```python
from build123d import *

# Parameters (mm, degrees)
SKETCH1_R           = 4.5
BOSS_EXTRUDE1_DEPTH = 2.4
SKETCH2_R           = 0.5
CUT_EXTRUDE1_DEPTH  = 0.5


with BuildPart() as part:
    # Sketch1 → Boss-Extrude1 (new body)
    with BuildSketch(Plane.XY):
        Circle(SKETCH1_R)
    extrude(amount=BOSS_EXTRUDE1_DEPTH)

    # Sketch2 → Cut-Extrude1 (cut)
    with BuildSketch(Plane(origin=(0, 0, 0), x_dir=(-1, 0, 0), z_dir=(0, 0, -1))):
        with Locations((2, 0.068183801)):
            Circle(SKETCH2_R)
        with Locations((-2, -0.055218249)):
            Circle(SKETCH2_R)
    extrude(amount=-CUT_EXTRUDE1_DEPTH, mode=Mode.SUBTRACT)


solid = part.part
```
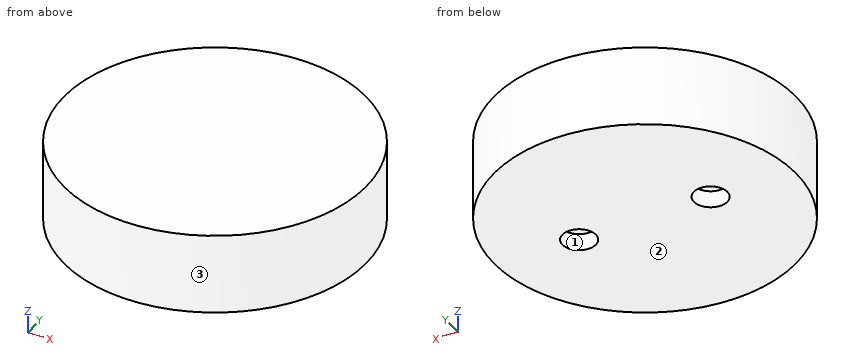
Read the model definition and answer for the solid it produces. Units are mm, in the model's axes. Face numbers are marked on the shaded views. Give positions to 0.01 mm unless a question says otherwise; leave off trailing zeros. Write each loop counter-clockwise with the first axis right and the second up, starting at its lowest first coordinate (ties: lowest second). Pieces come first, ordered by that corner, then holes. Notation, with made-up numbers: (74, -20) - (102, -20) arc R28 ccw to (102, 14) - close; hole circle Ø2 at (81.5, 1). An arc over 180 degrees is marked (long way). Write item = value, one per line. Start each with the question number.
Item 1: Find section D-D (z = 0.2). Give the vertices of the cut face in (x, y), then the cut area to 3 significant figures.
Item 2: Find section B-B (z = 1.7). Give the vertices of the cut face in (x, y).
Item 3: Find the intervals of material crossed by probe 1 along Y at (x, z) = (-2, 0.35); probe 2 along Z at (x, y) = (-1.75, 0); probe 3 along Y at (x, z) = (2, 0.4), in increasing order. Write a range as [from, to].
Item 4: Find section C-C (y = -0.25). Give the vertices of the cut face in (x, z), then the cut area to 3 significant figures.
Item 5: The mould has two halves that part along Y. Classify the marked faces 1, 2 and 3: +Y half, -Y half, draft (parallel to the pull), parting line (faces both ways), or undercut.
Item 6: Find section A-A (x = 2). Give the vertices of the cut face in (y, z), then the cut area to 3 significant figures.
Response:
q1.outline = circle Ø9 at (0, 0); hole circle Ø1 at (-2, 0.07); hole circle Ø1 at (2, -0.06)
q1.area = 62.0 mm²
q2.outline = circle Ø9 at (0, 0)
q3.probe_1 = [-4.03, -0.43], [0.57, 4.03]
q3.probe_2 = [0.5, 2.4]
q3.probe_3 = [-4.03, -0.56], [0.44, 4.03]
q4.outline = (-4.49, 0) - (-2.39, 0) - (-2.39, 0.5) - (-1.61, 0.5) - (-1.61, 0) - (1.54, 0) - (1.54, 0.5) - (2.46, 0.5) - (2.46, 0) - (4.49, 0) - (4.49, 2.4) - (-4.49, 2.4) - close
q4.area = 20.7 mm²
q5.face_1 = undercut
q5.face_2 = draft
q5.face_3 = parting line
q6.outline = (-4.03, 0) - (-0.56, 0) - (-0.56, 0.5) - (0.44, 0.5) - (0.44, 0) - (4.03, 0) - (4.03, 2.4) - (-4.03, 2.4) - close
q6.area = 18.8 mm²
